Verification items for the finished model (mm, model axes). Face numbers are marked on the shaded views. Give positions to 0.01 mm unless a question says otherwise; leave off trailing zeros. Loops run counter-clockwise (first coordinate to the right, second up) from the corner with the lowest first, then second, coordinate; pieces in that order, holes last. Notation, with made-up numbers: (-11.5, 71.5) - (-4.5, 71.5) arc R26 ccw to (-4.5, 86.5) - close; hole circle Ø10 at (-14.75, 55). An arc over 180 degrees is marked (long way). Put each result on its own line as item: value. Start each with the question number.
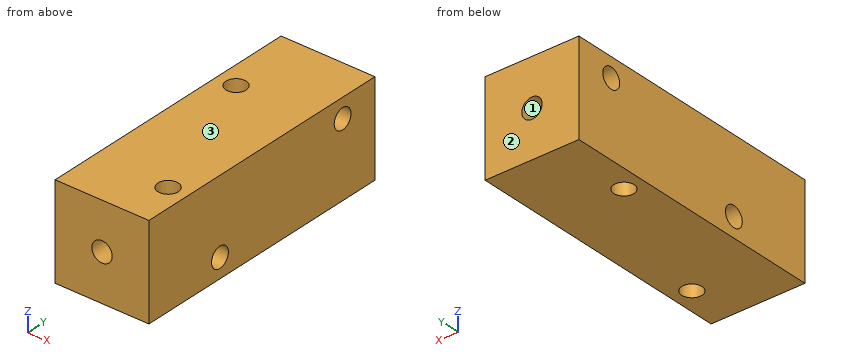
```python
from build123d import *

# Parameters (mm, degrees)
CYLINDER024_R           = 1.3
CYLINDER024_DEPTH       = 40
CYLINDER024_PITCH_ANGLE = 90
CYLINDER023_R           = 1.3
CYLINDER023_DEPTH       = 40
CYLINDER023_PITCH_ANGLE = 90
CYLINDER022_R           = 1.3
CYLINDER022_DEPTH       = 70
CYLINDER022_ROLL_ANGLE  = 90
CYLINDER021_R           = 1.3
CYLINDER021_DEPTH       = 40
CYLINDER020_R           = 1.3
CYLINDER020_DEPTH       = 40
BOX017_W                = 12
BOX017_H                = 35
BOX017_DEPTH            = 12


with BuildPart() as cylinder105:
    # Cylinder024 → Cylinder024 (new body)
    with BuildSketch(Plane.XY):
        Circle(CYLINDER024_R)
    extrude(amount=CYLINDER024_DEPTH)


with BuildPart() as cylinder105_1:
    # Cylinder024 pitch: moved
    add(cylinder105.part.rotate(Axis((0, 0, 0), (0, 1, 0)), CYLINDER024_PITCH_ANGLE))


with BuildPart() as cylinder105_2:
    # Cylinder024 placement: moved
    add(cylinder105_1.part.moved(Location((-40, 12, 9.5))))


with BuildPart() as fusion007:
    # Cylinder023 → Cylinder023 (new body)
    with BuildSketch(Plane.XY):
        Circle(CYLINDER023_R)
    extrude(amount=CYLINDER023_DEPTH)


with BuildPart() as fusion007_1:
    # Cylinder023 pitch: moved
    add(fusion007.part.rotate(Axis((0, 0, 0), (0, 1, 0)), CYLINDER023_PITCH_ANGLE))


with BuildPart() as fusion007_2:
    # Cylinder023 placement: moved
    add(fusion007_1.part.moved(Location((-40, -7, 2.5))))

    # Fusion007: union Cylinder105
    add(cylinder105_2.part)


with BuildPart() as fusion008:
    # Cylinder022 → Cylinder022 (new body)
    with BuildSketch(Plane.XY):
        Circle(CYLINDER022_R)
    extrude(amount=CYLINDER022_DEPTH)


with BuildPart() as fusion008_1:
    # Cylinder022 roll: moved
    add(fusion008.part.rotate(Axis((0, 0, 0), (1, 0, 0)), CYLINDER022_ROLL_ANGLE))


with BuildPart() as fusion008_2:
    # Cylinder022 placement: moved
    add(fusion008_1.part.moved(Location((-24, 39, 6))))

    # Fusion008: union Fusion007
    add(fusion007_2.part)


with BuildPart() as fusion009:
    # Cylinder021 → Cylinder021 (new body)
    with BuildSketch(Plane(origin=(-27.5, 7, -15), x_dir=(1, 0, 0), z_dir=(0, 0, 1))):
        Circle(CYLINDER021_R)
    extrude(amount=CYLINDER021_DEPTH)

    # Fusion009: union Fusion008
    add(fusion008_2.part)


with BuildPart() as corner_block_holes:
    # Cylinder020 → Cylinder020 (new body)
    with BuildSketch(Plane(origin=(-20.5, -12, -15), x_dir=(1, 0, 0), z_dir=(0, 0, 1))):
        Circle(CYLINDER020_R)
    extrude(amount=CYLINDER020_DEPTH)

    # Fusion010: union Fusion009
    add(fusion009.part)


with BuildPart() as corner_block002:
    # Box017 → Box017 (new body)
    with BuildSketch(Plane(origin=(-30, -18, 0), x_dir=(1, 0, 0), z_dir=(0, 0, 1))):
        with Locations((6, 17.5)):
            Rectangle(BOX017_W, BOX017_H)
    extrude(amount=BOX017_DEPTH)

    # Cut010: cut corner-block-holes
    add(corner_block_holes.part, mode=Mode.SUBTRACT)


with BuildPart() as corner_block002_1:
    # Cut010 placement: moved
    add(corner_block002.part.moved(Location((0, 0, 132))))


solid = corner_block002_1.part
```
1) Depth check by flat-ended pin: P1, Ø4, axis at y = 12, z = 141.5, coming from the -X side. Enter the tip coordinate at first touch or a pass-through.
2) Draft check along Z on the marked faces 1, 2 and 3. Enter one of: pulls with the +Z half, pulls with the -Z half, needs draft (parallel to the pull), parting line crosses it, or undercut.
3) Section check D-D, the plane y = 7. Enter the section's corners in (x, z), plus the area to 3 significant figures.
4) Scan lines: line 1 along Y through (x, z) = (-27.5, 134.5); line 2 along Y through (x, z) = (-21.5, 134); line 3 along Y through (x, z) = (-25, 134.5). Record each from-to range of solid material in increasing order. Write a range as from..to.
5) Section check C-C, the plane x = -27.5. Enter the section's corners in (y, z).
6) Section check B-B, the plane z = 141.5. Enter the section's corners in (x, y), plus the area to 3 significant figures.
7) Section check A-A, the plane y = -12.5. Enter the section's corners in (x, z), plus the area to 3 significant figures.
Results are:
1. P1: stops at x = -30
2. face 1: undercut
2. face 2: needs draft
2. face 3: pulls with the +Z half
3. outline: (-30, 132) - (-28.8, 132) - (-28.8, 144) - (-30, 144) - close; (-26.2, 132) - (-18, 132) - (-18, 144) - (-26.2, 144) - close; hole circle Ø2.6 at (-24, 138)
3. area: 107 mm2
4. line 1: y = -18..-8.3, -5.7..5.7, 8.3..17
4. line 2: y = -18..-12.83, -11.17..-8.2, -5.8..17
4. line 3: y = -18..-8.3, -5.7..17
5. outline: (-18, 132) - (5.7, 132) - (5.7, 144) - (-18, 144) - close; (8.3, 132) - (17, 132) - (17, 144) - (8.3, 144) - close; hole circle Ø2.6 at (-7, 134.5); hole circle Ø2.6 at (12, 141.5)
6. outline: (-30, -18) - (-18, -18) - (-18, 10.7) - (-30, 10.7) - close; (-30, 13.3) - (-18, 13.3) - (-18, 17) - (-30, 17) - close; hole circle Ø2.6 at (-27.5, 7); hole circle Ø2.6 at (-20.5, -12)
6. area: 378 mm2
7. outline: (-30, 132) - (-21.7, 132) - (-21.7, 144) - (-30, 144) - close; (-19.3, 132) - (-18, 132) - (-18, 144) - (-19.3, 144) - close; hole circle Ø2.6 at (-24, 138)
7. area: 110 mm2
